```python
from build123d import *

# Parameters (mm, degrees)
BOSS_EXTRUDE1_DEPTH = 3.048
SKETCH2_W           = 3.556
SKETCH2_H           = 6.858
CUT_EXTRUDE1_DEPTH  = 454.766547869


with BuildPart() as part:
    # Sketch1 → Boss-Extrude1 (new body)
    with BuildSketch(Plane.XY):
        with BuildLine():
            Line((-435.5719, 0), (-432.5239, 0))
            Line((-432.5239, 0), (-432.5239, -6.35))
            Line((-432.5239, -6.35), (-432.5239, -12.7))
            Line((-432.5239, -12.7), (-432.5239, -14.605))
            ThreePointArc((-432.5239, -14.605), (-434.197784746, -18.646115254), (-438.2389, -20.32))
            Line((-438.2389, -20.32), (-447.5861, -20.32))
            ThreePointArc((-447.5861, -20.32), (-451.627215254, -18.646115254), (-453.3011, -14.605))
            Line((-453.3011, -14.605), (-453.3011, -12.7))
            Line((-453.3011, -12.7), (-453.3011, -6.35))
            Line((-453.3011, -6.35), (-453.3011, 0))
            Line((-453.3011, 0), (-450.2531, 0))
            Line((-450.2531, 0), (-435.5719, 0))
        make_face()
    extrude(amount=BOSS_EXTRUDE1_DEPTH)

    # Sketch2 → Cut-Extrude1 (cut, through all)
    with BuildSketch(Plane.XY.offset(3.048)):
        with Locations((-434.0479, -9.525)):
            Rectangle(SKETCH2_W, SKETCH2_H)
        with Locations((-451.7771, -9.525)):
            Rectangle(SKETCH2_W, SKETCH2_H)
    extrude(amount=-CUT_EXTRUDE1_DEPTH, mode=Mode.SUBTRACT)


solid = part.part
```
Here's how the part is built. I have some questions about the finished solid (model axes, mm). A direction names the side the tool comes from. Coordinates: 2 decimals unless noted, no trailing zeros. Order: outer loops, then holes, each group sorted by start corner. A loop starts at its lowest first (then second) coordinate and runs counter-clockwise, first axis right, second up. Notation, with made-up numbers: (51, -14.5) - (61, -14.5) arc R17 cw to (61, 3.5) - close; hole circle Ø11 at (-8, -37). An arc over 180 degrees is marked (long way). One line per question, with ' | ' between items. Start each with the question number.
1. If we mould it in two halves opening along Y, with no side actions, what happens to faces 1 (the flat face through (-443, 0, 2)), 2 (the flat face through (-449.999, -10, 2)), 3 (the flat face through (-443, -10, 0)), 4 (the flat face through (-434, -12.954, 2))? For each: released by +Y, released by -Y, zero draft, split by the parting line, or undercut.
2. If we section it at B-B (y = -9): Write out the boundary of the cut face in (x, z).
3. If we section it at C-C (y = -18): Write out the boundary of the cut face in (x, z).
4. Which directions (+Z, -Z, +X, -X, +Y, -Y) give clear straight access to the entire face, cutting with the end or side of a thin tool? Please do faces 5 (the flat face through (-435.826, -10, 2)), 6 (the flat face through (-443, -10, 3.048)), 7 (the flat face through (-452, -12.954, 2)).
5. I'm going to push flat-ended pins straight in: pin 1 Ø3 at (x, y) = (-447.5, -11) entering from -Z; pin 2 Ø0.9 at (y, z) = (-10.5, 2) entering from -X; pin 3 Ø0.9 at (x, z) = (-434, 1) entering from -Y; pin 4 Ø1 at (y, z) = (-16, 0.5) entering from +X. Where does each tip first touch, or does it pass through?
6. Please list where these lines run through material, in increasing order: line 1 along X through (y, z) = (-7.75, 0.15); line 2 along X through (y, z) = (-14.75, 0.8); line 3 along Y through (x, z) = (-435.5, 1.75). Write a range as [from, to].
7. If we section it at A-A (z = 2.65): Write out the boundary of the cut face in (x, y) (3 decimals), and give its area (3 significant figures).
Model answer:
1) face 1: released by +Y | face 2: undercut | face 3: zero draft | face 4: undercut
2) outline: (-450, 0) - (-435.83, 0) - (-435.83, 3.05) - (-450, 3.05) - close
3) outline: (-452.18, 0) - (-433.64, 0) - (-433.64, 3.05) - (-452.18, 3.05) - close
4) face 5: +Z, -Z, +X | face 6: +Z, +X, -X, +Y, -Y | face 7: +Z, -Z, -X
5) pin 1: stops at z = 0 | pin 2: stops at x = -450 | pin 3: stops at y = -18.88 | pin 4: stops at x = -432.59
6) line 1: x = [-450, -435.83] | line 2: x = [-453.3, -432.53] | line 3: y = [-19.62, -12.95], [-6.1, 0]
7) outline: (-453.301, -14.605) arc R5.715 ccw to (-447.586, -20.32) - (-438.239, -20.32) arc R5.715 ccw to (-432.524, -14.605) - (-432.524, -12.954) - (-435.826, -12.954) - (-435.826, -6.096) - (-432.524, -6.096) - (-432.524, 0) - (-453.301, 0) - (-453.301, -6.096) - (-449.999, -6.096) - (-449.999, -12.954) - (-453.301, -12.954) - close | area: 363 mm²
